Geometry check sheet. Reference: the model listing, model coordinates, mm. Face numbers are marked on the shaded views. A direction names the side the tool comes from. Round coordinates to 2 decimals unless told otherwise and drop trailing zeros. Loops run counter-clockwise (first coordinate to the right, second up) from the corner with the lowest first, then second, coordinate; pieces in that order, holes last. Notation, with made-up numbers: (-33, 5.25) -> (-22, 5.25) arc R15 ccw to (-22, 19.25) -> close; hole circle Ø4 at (-34, -37.75). An arc over 180 degrees is marked (long way). Use a Markdown table: item, result. Add a question column.
Q1. Material ranges on L1, parallel to X at y = -17, z = 23.5; L2, parallel to Y at x = 9, z = 7 (3 decimals); L3, parallel to Z at x = -10, y = 21, recorded low to high.
Q2. Sectioned sample at A-A, the plane y = 1. Enter the section's corners in (x, z) (3 decimals).
Q3. Release check for a two-part mould opening along X. For the marked faces 4, 5 and 6 record: released by +X, released by -X, zero draft, split by the parting line, or undercut.
Q4. Set-up check for the marked faces 1, 2 and 3: record each of +Z, -Z, +X, -X, +Y, -Y from which the full face is reachable in a straight line by a thin tool's end or side.
Q5. Sectioned sample at B-B, the plane x = -28. Enter the section's corners in (y, z), then the cut area to 4 significant figures.
Q6. Gauge pin test, flat ends, axial feed: P1, Ø10, axis at x = 15, y = 26.5, coming from the +Z side; P2, Ø13, axis at x = 11, z = 28, coming from the -Y side; P3, Ø1.1, axis at x = 25.5, y = -25, coming from the -Z side. Record the tip position at first contact, or that the pin passes through.
Q7. Sectioned sample at D-D, the plane y = -10. Enter the section's corners in (x, z) (3 decimals), then the cut area to 3 significant figures.
Q8. Sectioned sample at C-C, the plane z = 8. Enter the section's corners in (x, y) (3 decimals).
```python
from build123d import *

# Parameters (mm, degrees)
SKETCH1_W               = 60
SKETCH1_H               = 51
BOSS_EXTRUDE3_DEPTH     = 48
CUT_EXTRUDE1_DEPTH      = 18
CUT_EXTRUDE2_DEPTH      = 77.190550595
CUT_EXTRUDE2_DEPTH_BACK = 11.25
SKETCH2_W               = 40
SKETCH2_H               = 18
BOSS_EXTRUDE4_DEPTH     = 30
FILLET1_R               = 8
SHELL1_T                = -1
CUT_EXTRUDE5_START      = -1
CUT_EXTRUDE5_DEPTH      = 1
SKETCH5_W               = 6
SKETCH5_H               = 9
CUT_EXTRUDE4_DEPTH      = 1


# Read off the part's stored shape, not the designer's step: Cut-Extrude5
with BuildPart() as part:
    # Sketch1 → Boss-Extrude3 (new body)
    with BuildSketch(Plane(origin=(0, 0, 0), x_dir=(-1, 0, 0), z_dir=(0, 0, -1))):
        Rectangle(SKETCH1_W, SKETCH1_H)
    extrude(amount=-BOSS_EXTRUDE3_DEPTH)

    # Sketch1<6> → Cut-Extrude1 (cut)
    with BuildSketch(Plane(origin=(0, 0, 0), x_dir=(-1, 0, 0), z_dir=(0, 0, -1))):
        Polygon((-20, -25.5), (-20, -14.25), (20, -14.25), (20, -25.5), (30, -25.5), (30, 25.5), (-30, 25.5), (-30, -25.5), align=None)
        Polygon((21.375, -12.625), (-21.375, -12.625), (-21.375, -6.75), (-28.375, -6.75), (-28.375, 4.25), (-21.375, 4.25), (-21.375, 10.125), (21.375, 10.125), align=None, mode=Mode.SUBTRACT)
    extrude(amount=-CUT_EXTRUDE1_DEPTH, mode=Mode.SUBTRACT)

    # Sketch2 → Cut-Extrude2 (cut, two sides: drawn at the far end of the back side and taken through both)
    with BuildSketch(Plane.XZ.offset(25.5).offset(-CUT_EXTRUDE2_DEPTH_BACK)):
        with Locations((0, 9)):
            Rectangle(SKETCH2_W, SKETCH2_H)
    extrude(amount=CUT_EXTRUDE2_DEPTH + CUT_EXTRUDE2_DEPTH_BACK, mode=Mode.SUBTRACT)

    # Sketch6 → Boss-Extrude4 (add)
    with BuildSketch(Plane.XY.offset(48)):
        Polygon((30, 25.5), (30, -25.5), (32, -25.5), (32, 34.5), (-39, 34.5), (-39, -25.5), (-30, -25.5), (-30, 25.5), align=None)
    extrude(amount=-BOSS_EXTRUDE4_DEPTH)

    # Fillet1
    fillet1_edges = [part.edges().sort_by_distance(p)[0] for p in [
        (-39, 34.5, 33),
        (32, 34.5, 33),
        (32, -25.5, 33),
        (-39, -25.5, 33),
    ]]
    fillet(fillet1_edges, radius=FILLET1_R)

    # Shell1
    shell1_openings = [part.faces().sort_by_distance(p)[0] for p in [
        (-3.5, 4.5, 48),
    ]]
    offset(amount=SHELL1_T, openings=shell1_openings, kind=Kind.INTERSECTION)

    # Cut-Extrude5 outline → Cut-Extrude5 (cut)
    with BuildSketch(Plane.XZ.offset(25.5).offset(CUT_EXTRUDE5_START)):
        with BuildLine():
            Line((29, 44.25), (20, 44.25))
            ThreePointArc((20, 44.25), (19.911125548, 46.13336917), (19.645292057, 48))
            Line((19.645292057, 48), (-19.645292057, 48))
            ThreePointArc((-19.645292057, 48), (-19.911125548, 46.13336917), (-20, 44.25))
            Line((-20, 44.25), (-30, 44.25))
            Line((-30, 44.25), (-30, 17))
            Line((-30, 17), (29, 17))
            Line((29, 17), (29, 44.25))
        make_face()
    extrude(amount=CUT_EXTRUDE5_DEPTH, mode=Mode.SUBTRACT)

    # Sketch5 → Cut-Extrude4 (cut)
    with BuildSketch(Plane(origin=(28.375, 0, 0), x_dir=(0, 0, -1), z_dir=(1, 0, 0))):
        with Locations((-6, -1.25)):
            Rectangle(SKETCH5_W, SKETCH5_H)
    extrude(amount=-CUT_EXTRUDE4_DEPTH, mode=Mode.SUBTRACT)


solid = part.part
```
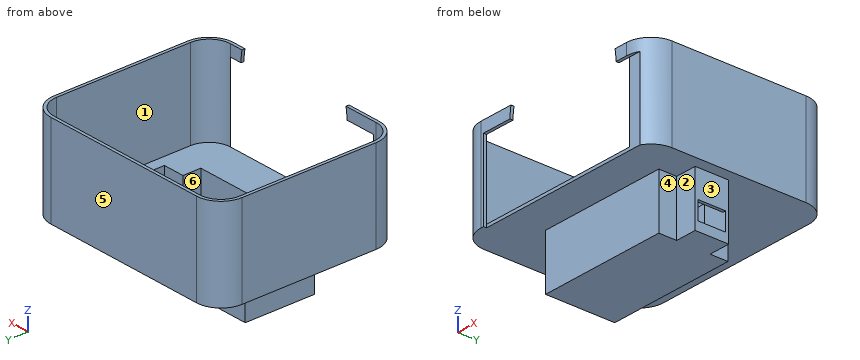
Values:
| question | item | result |
|---|---|---|
| 1 | L1 | -39 to -38, 31 to 32 |
| 1 | L2 | -12.625 to -11.625, 9.125 to 10.125 |
| 1 | L3 | 18 to 19 |
| 2 | outline | (-39, 18) -> (-21.375, 18) -> (-21.375, 0) -> (28.375, 0) -> (28.375, 3) -> (27.375, 3) -> (27.375, 1) -> (-20.375, 1) -> (-20.375, 19) -> (-38, 19) -> (-38, 48) -> (-39, 48) -> close; (27.375, 9) -> (28.375, 9) -> (28.375, 18) -> (32, 18) -> (32, 48) -> (31, 48) -> (31, 19) -> (27.375, 19) -> close |
| 3 | face 4 | released by +X |
| 3 | face 5 | zero draft |
| 3 | face 6 | undercut |
| 4 | face 1 | +Z |
| 4 | face 2 | -Z, +X, -Y |
| 4 | face 3 | -Z, +X, +Y, -Y |
| 5 | outline | (-25.5, 44.25) -> (-24.5, 44.25) -> (-24.5, 48) -> (-25.5, 48) -> close; (-24.5, 18) -> (34.5, 18) -> (34.5, 48) -> (33.5, 48) -> (33.5, 19) -> (-24.5, 19) -> close |
| 5 | area | 91.75 mm^2 |
| 6 | P1 | z = 19 |
| 6 | P2 | y = 33.5 |
| 6 | P3 | z = 18 |
| 7 | outline | (-39, 18) -> (-21.375, 18) -> (-21.375, 0) -> (21.375, 0) -> (21.375, 18) -> (32, 18) -> (32, 48) -> (31, 48) -> (31, 19) -> (20.375, 19) -> (20.375, 1) -> (-20.375, 1) -> (-20.375, 19) -> (-38, 19) -> (-38, 48) -> (-39, 48) -> close |
| 7 | area | 165 mm^2 |
| 8 | outline | (-21.375, -12.625) -> (21.375, -12.625) -> (21.375, -6.75) -> (28.375, -6.75) -> (28.375, -5.75) -> (20.375, -5.75) -> (20.375, -11.625) -> (-20.375, -11.625) -> (-20.375, 9.125) -> (20.375, 9.125) -> (20.375, 3.25) -> (28.375, 3.25) -> (28.375, 4.25) -> (21.375, 4.25) -> (21.375, 10.125) -> (-21.375, 10.125) -> close |
